```python
from build123d import *

# Parameters (mm, degrees)
SKETCH1_W            = 22
SKETCH1_H            = 32
BOSS_EXTRUDE1_DEPTH  = 25.5
CUT_EXTRUDE1_START   = -4.8125
CUT_EXTRUDE1_DEPTH   = 15.75
CUT_EXTRUDE1_START_2 = 1.4375
CUT_EXTRUDE1_2_DEPTH = 9.5
SKETCH8_W            = 9.5
SKETCH8_H            = 26
BOSS_EXTRUDE2_DEPTH  = 25.5
CUT_EXTRUDE2_DEPTH   = 9.5
SKETCH10_W           = 12.5
SKETCH10_H           = 32
BOSS_EXTRUDE3_DEPTH  = 25.5
CUT_EXTRUDE3_START   = -17.3125
CUT_EXTRUDE3_DEPTH   = 12.5
FILLET1_R            = 8


# Read off the part's stored shape, not the designer's step: Cut-Extrude1, Cut-Extrude3
with BuildPart() as part:
    # Sketch1 → Boss-Extrude1 (new body)
    with BuildSketch(Plane.XY):
        with Locations((6.1875, -13.307291667)):
            Rectangle(SKETCH1_W, SKETCH1_H)
    extrude(amount=BOSS_EXTRUDE1_DEPTH)

    # Cut-Extrude1 outline → Cut-Extrude1 (cut)
    with BuildSketch(Plane.YZ.offset(CUT_EXTRUDE1_START)):
        Polygon((-29.307291667, 25.5), (-29.307291667, 16), (-14.609886779, 20.899134963), (-14.609886779, 25.5), align=None)
    extrude(amount=CUT_EXTRUDE1_DEPTH, mode=Mode.SUBTRACT)

    # Cut-Extrude1 2 outline → Cut-Extrude1 2 (cut)
    with BuildSketch(Plane.YZ.offset(CUT_EXTRUDE1_START_2)):
        Polygon((-14.609886779, 25.5), (-14.609886779, 20.899134963), (-0.807291667, 25.5), align=None)
    extrude(amount=CUT_EXTRUDE1_2_DEPTH, mode=Mode.SUBTRACT)

    # Sketch8 → Boss-Extrude2 (add)
    with BuildSketch(Plane.XY):
        with Locations((21.9375, -10.307291667)):
            Rectangle(SKETCH8_W, SKETCH8_H)
    extrude(amount=BOSS_EXTRUDE2_DEPTH)

    # Sketch9 → Cut-Extrude2 (cut)
    with BuildSketch(Plane(origin=(26.6875, 0, 0), x_dir=(0, 0, -1), z_dir=(1, 0, 0))):
        with BuildLine():
            Line((-18.837056558, -8.265810445), (-25.5, -0.807291667))
            Line((-25.5, -0.807291667), (-25.5, -23.307291667))
            Line((-25.5, -23.307291667), (-5.4, -23.307291667))
            Line((-5.4, -23.307291667), (-10.176291277, -17.960696954))
            ThreePointArc((-10.176291277, -17.960696954), (-19.347447848, -17.437678411), (-18.837056558, -8.265810445))
        make_face()
        with BuildLine():
            ThreePointArc((-8, -13.107291667), (-11.848667092, -7.172611068), (-18.837056558, -8.265810445))
            Line((-18.837056558, -8.265810445), (-10.176291277, -17.960696954))
            ThreePointArc((-10.176291277, -17.960696954), (-8.568975354, -15.76679287), (-8, -13.107291667))
        make_face()
        with BuildLine():
            Line((-10.176291277, -17.960696954), (-18.837056558, -8.265810445))
            ThreePointArc((-18.837056558, -8.265810445), (-19.347447848, -17.437678411), (-10.176291277, -17.960696954))
        make_face()
    extrude(amount=-CUT_EXTRUDE2_DEPTH, mode=Mode.SUBTRACT)

    # Sketch10 → Boss-Extrude3 (add)
    with BuildSketch(Plane.XY):
        with Locations((-11.0625, -13.307291667)):
            Rectangle(SKETCH10_W, SKETCH10_H)
    extrude(amount=BOSS_EXTRUDE3_DEPTH)

    # Cut-Extrude3 outline → Cut-Extrude3 (cut)
    with BuildSketch(Plane.YZ.offset(CUT_EXTRUDE3_START)):
        Polygon((-29.307291667, 9.5), (-0.807291667, 25.5), (-29.307291667, 25.5), align=None)
    extrude(amount=CUT_EXTRUDE3_DEPTH, mode=Mode.SUBTRACT)

    # Fillet1
    fillet1_edges = [part.edges().sort_by_distance(p)[0] for p in [
        (-17.3125, -29.307291667, 4.75),
    ]]
    fillet(fillet1_edges, radius=FILLET1_R)


solid = part.part
```
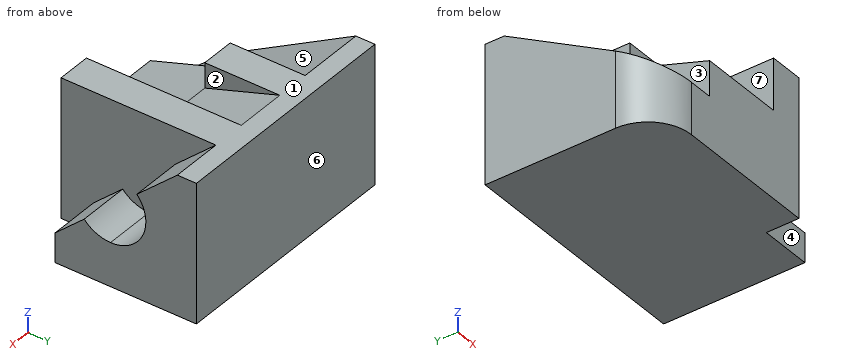
Here's how the part is built. I have some questions about the finished solid (model axes, mm). Face numbers are marked on the shaded views. A direction names the side the tool comes from. Coordinates: 2 decimals unless noted, no trailing zeros. Loops run counter-clockwise (first coordinate to the right, second up) from the corner with the lowest first, then second, coordinate; pieces in that order, holes last. Notation, with made-up numbers: (88, -19) - (98, -19) arc R13 cw to (98, -6) - close; hole circle Ø1 at (24.25, 63.5). An arc over 180 degrees is marked (long way). Return JSON: item names as keys, results as strings. Group by question number.
Item 1: If we section it at B-B on y = -5: Write out the boundary of the cut face in (x, z), and give its area (3 significant figures).
Item 2: I need wall thicknesses on line 1 (X direction, y = -11.5, z = 15.5); line 2 (X direction, y = -25, z = 17); line 3 (Z direction, x = 23, y = -13). Which ranges of each line are inside material? Lowest first, please. Write a range as from..to.
Item 3: On a 3-axis mill with a long thin cutter (end or side, diameter ignored), from which of +Z, -Z, +X, -X, +Y, -Y can I reach the whole of each face in a straight line? I mean the marked faces 4, 5, 6 and 7. Say none if no direction works.
Item 4: Will these pins go through, and if not, where does the flat tip stop? P1, Ø5, axis at y = -22, z = 17, coming from the -X side; P2, Ø5, axis at y = -8.5, z = 22.5, coming from the +X side; P3, Ø1.4, axis at x = -2, z = 24, coming from the -Y side.
Item 5: If we section it at A-A on x = -6: Write out the boundary of the cut face in (y, z), and give its area (3 significant figures).
Item 6: We'd pull the mould along X, two halves only. Please class the marked faces 1, 2 and 3: +X half, -X half, draft (parallel to the pull), parting line (faces both ways), or undercut.
Item 7: If we section it at C-C on z = 4.5: Write out the boundary of the cut face in (x, y).
Item 8: If we section it at D-D on y = -9: Write out the boundary of the cut face in (x, z).
Calculated:
{
 "1": {"outline": "(-17.31, 0) - (26.69, 0) - (26.69, 21.75) - (17.19, 21.75) - (17.19, 25.5) - (10.94, 25.5) - (10.94, 24.1) - (1.44, 24.1) - (1.44, 25.5) - (-4.81, 25.5) - (-4.81, 23.15) - (-17.31, 23.15) - close", "area": "1,040 mm^2"},
 "2": {"line 1": "x = -17.31..17.19", "line 2": "x = -4.81..17.19", "line 3": "z = 0..8"},
 "3": {"face 4": "+Z, -Z, +X, -Y", "face 5": "+Z, -X, -Y", "face 6": "+Z, -Z, +X, -X, +Y", "face 7": "+Z, -Y"},
 "4": {"P1": "stops at x = -4.81", "P2": "stops at x = 17.19", "P3": "stops at y = -14.61"},
 "5": {"outline": "(-29.31, 0) - (2.69, 0) - (2.69, 25.5) - (-0.81, 25.5) - (-29.31, 9.5) - close", "area": "588 mm^2"},
 "6": {"face 1": "draft", "face 2": "undercut", "face 3": "-X half"},
 "7": {"outline": "(-17.31, -21.31) arc R8 ccw to (-9.31, -29.31) - (17.19, -29.31) - (17.19, -23.31) - (26.69, -23.31) - (26.69, 2.69) - (-17.31, 2.69) - close"},
 "8": {"outline": "(-17.31, 0) - (26.69, 0) - (26.69, 9.46) - (17.19, 9.46) - (17.19, 25.5) - (10.94, 25.5) - (10.94, 22.77) - (1.44, 22.77) - (1.44, 25.5) - (-4.81, 25.5) - (-4.81, 20.9) - (-17.31, 20.9) - close"}
}
